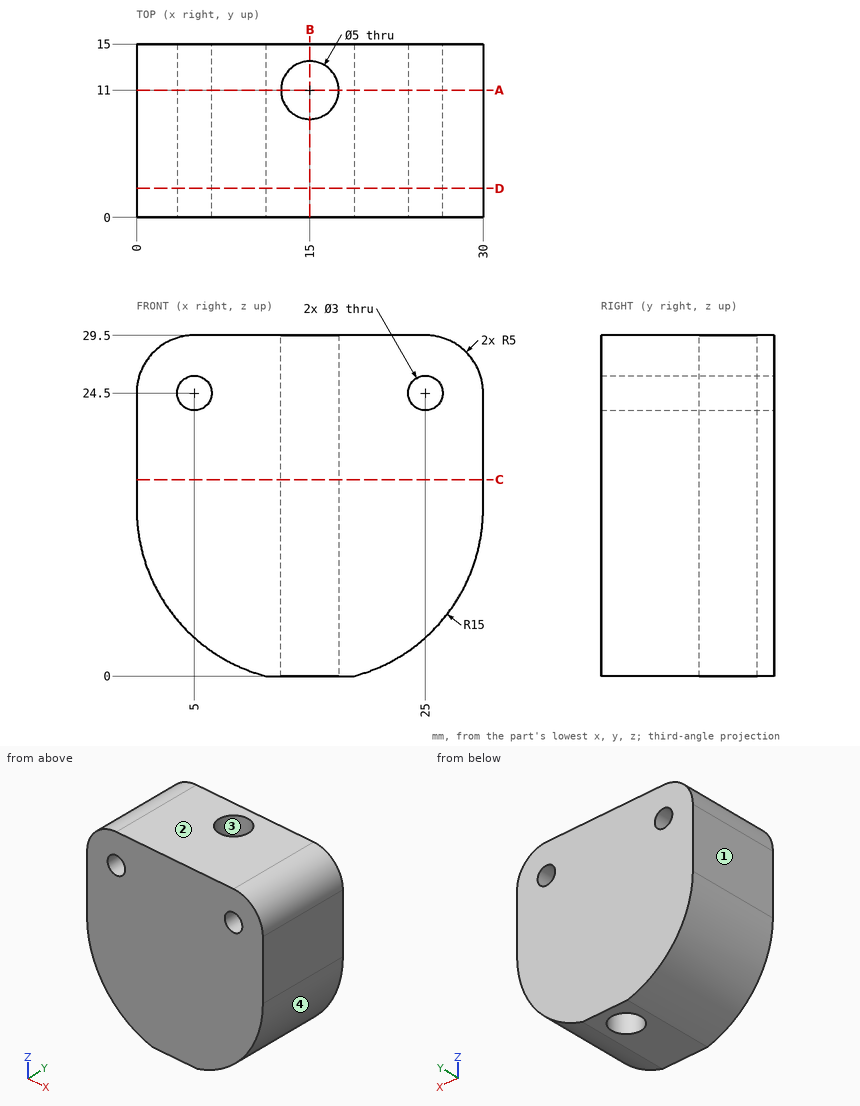
Design review of the part shown in the three views and the two pictorial views. Dimensions are in mm from the part's minimum x, y and z. Coordinates: 2 decimals unless noted, no trailing zeros. Order: outer loops, then holes, each group sorted by start corner. A loop starts at its lowest first (then second) coordinate and runs counter-clockwise, first axis right, second up. Notation, with made-up numbers: (38, -14) - (50, -14) arc R27 ccw to (50, 22) - close; hole circle Ø1 at (23.25, 79). An arc over 180 degrees is marked (long way). Answer as CSV lines item,"result". Start each with the question number.
1) Insertion check: P1, Ø8, axis at y = 8.5, z = 7, coming from the +X side; P2, Ø5, axis at y = 7.5, z = 9, coming from the +X side; P3, Ø8, axis at y = 12.5, z = 6, coming from the -X side. Each pin has a flat end and moves straight along its axis. Give the tip position at first contact, or say it passes through.
2) Add section A-A (y = 11). State the section outline as (x, z) points, then the cut area to 3 significant figures.
3) Add section D-D (y = 2.5). State the section outline as (x, z) points.
4) Add section B-B (x = 15). State the section outline as (y, z) points, then the cut area to 3 significant figures.
5) Draft analysis for pull direction X (two halves, no side actions). For the marked faces 1, 2, 3 and 4, state which applies: +X half, -X half, draft (parallel to the pull), parting line (faces both ways), or undercut.
6) Add section C-C (z = 17). State the section outline as (x, y) points.
7) To check wall thickness, follow line 1 along X through (y, z) = (6.5, 24.25); line 2 along Z through (x, y) = (5, 5.5); line 3 along Y through (x, z) = (13.25, 23.5). State the ranges of each line that lie inside material, in increasing order. Write a range as [from, to].
Result:
1,P1,"x = 29.59"
1,P2,"x = 29.7"
1,P3,"x = 0.69"
2,outline,"(0, 14.5) arc R15 ccw to (11.16, 0) - (12.5, 0) - (12.5, 29.5) - (5, 29.5) arc R5 ccw to (0, 24.5) - close; (17.5, 0) - (18.84, 0) arc R15 ccw to (30, 14.5) - (30, 24.5) arc R5 ccw to (25, 29.5) - (17.5, 29.5) - close; hole circle Ø3 at (5, 24.5); hole circle Ø3 at (25, 24.5)"
2,area,"628 mm^2"
3,outline,"(0, 14.5) arc R15 ccw to (11.16, 0) - (18.84, 0) arc R15 ccw to (30, 14.5) - (30, 24.5) arc R5 ccw to (25, 29.5) - (5, 29.5) arc R5 ccw to (0, 24.5) - close; hole circle Ø3 at (5, 24.5); hole circle Ø3 at (25, 24.5)"
4,outline,"(0, 0) - (8.5, 0) - (8.5, 29.5) - (0, 29.5) - close; (13.5, 0) - (15, 0) - (15, 29.5) - (13.5, 29.5) - close"
4,area,"295 mm^2"
5,face 1,"-X half"
5,face 2,"draft"
5,face 3,"undercut"
5,face 4,"+X half"
6,outline,"(0, 0) - (30, 0) - (30, 15) - (0, 15) - close; hole circle Ø5 at (15, 11)"
7,line 1,"[0, 3.52], [6.48, 23.52], [26.48, 30]"
7,line 2,"[3.32, 23], [26, 29.5]"
7,line 3,"[0, 9.21], [12.79, 15]"
